Verification items for the finished model (mm, model axes). Round coordinates to 2 decimals unless told otherwise and drop trailing zeros. Write each loop counter-clockwise with the first axis right and the second up, starting at its lowest first coordinate (ties: lowest second). Pieces come first, ordered by that corner, then holes. Notation, with made-up numbers: (-25, -25.5) - (18, -25.5) arc R15 ccw to (18, 1.5) - close; hole circle Ø6 at (67, -38). An arc over 180 degrees is marked (long way). Answer as a JSON object with one key per item and string values. Group by question number.
1) Thickness scan on line 1 (X direction, y = 0.15, z = -14.5); line 2 (X direction, y = 0.45, z = -32); line 3 (Z direction, x = 1.5, y = 0.2). Record the ranges inside material, lowest first.
2) Section check D-D (x = 9). Enter the section's corners in (y, z).
3) Mould release check, pull along X, two halves, no side actions. Record for faces 1 (the flat face through (15.9, 0.5, -29.4)), 2 (the cylindrical face through (13.6, 0.2, -33.2)): +X half, -X half, draft (parallel to the pull), parting line (faces both ways), or undercut.
4) Section check C-C (z = 3). Enter the section's corners in (x, y), then the cut area to 3 significant figures.
5) Section check B-B (y = 0.1). State how many separate pieces and enclosed holes the cut face has, then the cut area to 3 significant figures.
6) Section check A-A (z = -2). Enter the section's corners in (x, y).
```python
from build123d import *

# Parameters (mm, degrees)
CROQUIS1_R              = 1.5
CROQUIS1_W              = 29
CROQUIS1_H              = 29
SALIENTE_EXTRUIR1_DEPTH = 0.5


with BuildPart() as part:
    # Croquis1 → Saliente-Extruir1 (new body)
    with BuildSketch(Plane(origin=(0, 0, 0), x_dir=(1, 0, 0), z_dir=(0, 1, 0))):
        with BuildLine():
            ThreePointArc((-5.5, -5.381384118), (-5.449888151, -5.441258419), (-5.398453182, -5.5))
            Line((-5.398453182, -5.5), (34.5, -5.5))
            Line((34.5, -5.5), (34.5, 34.5))
            Line((34.5, 34.5), (-5.5, 34.5))
            Line((-5.5, 34.5), (-5.5, -5.381384118))
        make_face()
        with Locations(Location((6.5, -3, 0), (0, 0, 270))):
            Circle(CROQUIS1_R, mode=Mode.SUBTRACT)
        with Locations(Location((-3, 6.5, 0), (0, 0, 270))):
            Circle(CROQUIS1_R, mode=Mode.SUBTRACT)
        with Locations((14.5, 14.5)):
            Rectangle(CROQUIS1_W, CROQUIS1_H, mode=Mode.SUBTRACT)
        with Locations(Location((14.5, -3, 0), (0, 0, 270))):
            Circle(CROQUIS1_R, mode=Mode.SUBTRACT)
        with Locations(Location((22.5, -3, 0), (0, 0, 270))):
            Circle(CROQUIS1_R, mode=Mode.SUBTRACT)
        with Locations(Location((32, 6.5, 0), (0, 0, 270))):
            Circle(CROQUIS1_R, mode=Mode.SUBTRACT)
        with Locations(Location((32, 14.5, 0), (0, 0, 270))):
            Circle(CROQUIS1_R, mode=Mode.SUBTRACT)
        with Locations(Location((-3, 14.5, 0), (0, 0, 270))):
            Circle(CROQUIS1_R, mode=Mode.SUBTRACT)
        with Locations(Location((-3, 22.5, 0), (0, 0, 270))):
            Circle(CROQUIS1_R, mode=Mode.SUBTRACT)
        with Locations(Location((6.5, 32, 0), (0, 0, 270))):
            Circle(CROQUIS1_R, mode=Mode.SUBTRACT)
        with Locations(Location((32, 22.5, 0), (0, 0, 270))):
            Circle(CROQUIS1_R, mode=Mode.SUBTRACT)
        with Locations(Location((14.5, 32, 0), (0, 0, 270))):
            Circle(CROQUIS1_R, mode=Mode.SUBTRACT)
        with Locations(Location((22.5, 32, 0), (0, 0, 270))):
            Circle(CROQUIS1_R, mode=Mode.SUBTRACT)
    extrude(amount=SALIENTE_EXTRUIR1_DEPTH)


solid = part.part
```
Returned:
{
 "1": {"line 1": "-5.5 to -4.5, -1.5 to 0, 29 to 30.5, 33.5 to 34.5", "line 2": "-5.5 to 5, 8 to 13, 16 to 21, 24 to 34.5", "line 3": "-34.5 to -29, 0 to 5.5"},
 "2": {"outline": "(0, -34.5) - (0.5, -34.5) - (0.5, -29) - (0, -29) - close; (0, 0) - (0.5, 0) - (0.5, 5.5) - (0, 5.5) - close"},
 "3": {"face 1": "draft", "face 2": "undercut"},
 "4": {"outline": "(-5.5, 0) - (5, 0) - (5, 0.5) - (-5.5, 0.5) - close; (8, 0) - (13, 0) - (13, 0.5) - (8, 0.5) - close; (16, 0) - (21, 0) - (21, 0.5) - (16, 0.5) - close; (24, 0) - (34.5, 0) - (34.5, 0.5) - (24, 0.5) - close", "area": "15.5 mm2"},
 "5": {"separate pieces": "1", "enclosed holes": "13", "area": "674 mm2"},
 "6": {"outline": "(-5.5, 0) - (0, 0) - (0, 0.5) - (-5.5, 0.5) - close; (29, 0) - (34.5, 0) - (34.5, 0.5) - (29, 0.5) - close"}
}
